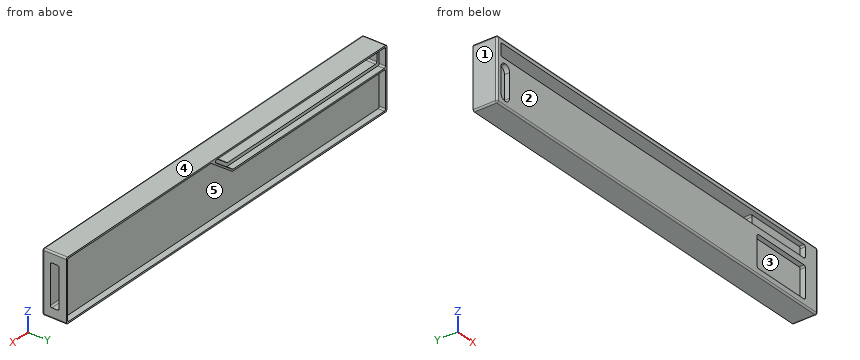
```python
from build123d import *

# Parameters (mm, degrees)
EXTRUDE_1_DEPTH     = 7.6
CUT_EXTRUDE_1_DEPTH = 2
CUT_EXTRUDE_2_DEPTH = 66.965312855
CUT_EXTRUDE_START   = -1.6
CUT_EXTRUDE_3_DEPTH = 1.6
CUT_EXTRUDE_START_2 = -3.3
CUT_EXTRUDE_4_DEPTH = 3.3
CUT_EXTRUDE_5_DEPTH = 10
FILLET_1_R          = 0.5


with BuildPart() as part:
    # Эскиз1 → Бобышка-Вытянуть1 (new body)
    with BuildSketch(Plane(origin=(0, 0, 0), x_dir=(1, 0, 0), z_dir=(0, 1, 0))):
        with BuildLine():
            Line((-64.5, 9.75), (64.5, 9.75))
            ThreePointArc((64.5, 9.75), (64.853553391, 9.603553391), (65, 9.25))
            Line((65, 9.25), (65, -9.25))
            ThreePointArc((65, -9.25), (64.853553391, -9.603553391), (64.5, -9.75))
            Line((64.5, -9.75), (-64.5, -9.75))
            ThreePointArc((-64.5, -9.75), (-64.853553391, -9.603553391), (-65, -9.25))
            Line((-65, -9.25), (-65, 9.25))
            ThreePointArc((-65, 9.25), (-64.853553391, 9.603553391), (-64.5, 9.75))
        make_face()
    extrude(amount=EXTRUDE_1_DEPTH)

    # Эскиз2 → Вырез-Вытянуть1 (cut)
    with BuildSketch(Plane(origin=(0, 7.6, 0), x_dir=(1, 0, 0), z_dir=(0, 1, 0))):
        with BuildLine():
            Line((-64, -3.25), (-2.666666667, -3.25))
            ThreePointArc((-2.666666667, -3.25), (-2.508552784, -3.275658351), (-2.366666667, -3.35))
            Line((-2.366666667, -3.35), (4.3, -8.35))
            ThreePointArc((4.3, -8.35), (4.474341649, -8.908113883), (4, -9.25))
            Line((4, -9.25), (-64, -9.25))
            ThreePointArc((-64, -9.25), (-64.353553391, -9.103553391), (-64.5, -8.75))
            Line((-64.5, -8.75), (-64.5, -3.75))
            ThreePointArc((-64.5, -3.75), (-64.353553391, -3.396446609), (-64, -3.25))
        make_face()
        with BuildLine():
            Line((-64, 9.25), (64, 9.25))
            ThreePointArc((64, 9.25), (64.353553391, 9.103553391), (64.5, 8.75))
            Line((64.5, 8.75), (64.5, -8.75))
            ThreePointArc((64.5, -8.75), (64.353553391, -9.103553391), (64, -9.25))
            Line((64, -9.25), (6.5, -9.25))
            ThreePointArc((6.5, -9.25), (6.341886117, -9.224341649), (6.2, -9.15))
            Line((6.2, -9.15), (-2.2, -2.85))
            ThreePointArc((-2.2, -2.85), (-2.341886117, -2.775658351), (-2.5, -2.75))
            Line((-2.5, -2.75), (-64, -2.75))
            ThreePointArc((-64, -2.75), (-64.353553391, -2.603553391), (-64.5, -2.25))
            Line((-64.5, -2.25), (-64.5, 8.75))
            ThreePointArc((-64.5, 8.75), (-64.353553391, 9.103553391), (-64, 9.25))
        make_face()
    extrude(amount=-CUT_EXTRUDE_1_DEPTH, mode=Mode.SUBTRACT)

    # Эскиз6 → Вырез-Вытянуть2 (cut, through all)
    with BuildSketch(Plane(origin=(0, 5.6, 0), x_dir=(1, 0, 0), z_dir=(0, 1, 0))):
        with BuildLine():
            Line((-63, -8.25), (1.020582083, -8.25))
            ThreePointArc((1.020582083, -8.25), (1.494923732, -7.908113883), (1.320582083, -7.35))
            Line((1.320582083, -7.35), (-2.695152274, -4.338199232))
            ThreePointArc((-2.695152274, -4.338199232), (-2.837038391, -4.263857583), (-2.995152274, -4.238199232))
            Line((-2.995152274, -4.238199232), (-63, -4.238199232))
            ThreePointArc((-63, -4.238199232), (-63.353553391, -4.384645841), (-63.5, -4.738199232))
            Line((-63.5, -4.738199232), (-63.5, -7.75))
            ThreePointArc((-63.5, -7.75), (-63.353553391, -8.103553391), (-63, -8.25))
        make_face()
    extrude(amount=-CUT_EXTRUDE_2_DEPTH, mode=Mode.SUBTRACT)

    # Эскиз7 → Вырез-Вытянуть3 (cut)
    with BuildSketch(Plane.XZ.offset(CUT_EXTRUDE_START)):
        with BuildLine():
            Line((-63, 4.25), (59.5, 4.25))
            ThreePointArc((59.5, 4.25), (59.853553391, 4.396446609), (60, 4.75))
            Line((60, 4.75), (60, 7.75))
            ThreePointArc((60, 7.75), (59.853553391, 8.103553391), (59.5, 8.25))
            Line((59.5, 8.25), (-63, 8.25))
            ThreePointArc((-63, 8.25), (-63.353553391, 8.103553391), (-63.5, 7.75))
            Line((-63.5, 7.75), (-63.5, 4.75))
            ThreePointArc((-63.5, 4.75), (-63.353553391, 4.396446609), (-63, 4.25))
        make_face()
        with BuildLine():
            Line((59.5, -7.75), (41, -7.75))
            ThreePointArc((41, -7.75), (40.646446609, -7.603553391), (40.5, -7.25))
            Line((40.5, -7.25), (40.5, 1.75))
            ThreePointArc((40.5, 1.75), (40.646446609, 2.103553391), (41, 2.25))
            Line((41, 2.25), (59.5, 2.25))
            ThreePointArc((59.5, 2.25), (59.853553391, 2.103553391), (60, 1.75))
            Line((60, 1.75), (60, -7.25))
            ThreePointArc((60, -7.25), (59.853553391, -7.603553391), (59.5, -7.75))
        make_face()
        with BuildLine():
            Line((-61.74, -8.15), (-61.76, -8.15))
            ThreePointArc((-61.76, -8.15), (-62.990365799, -7.640365799), (-63.5, -6.41))
            Line((-63.5, -6.41), (-63.5, 1.11))
            ThreePointArc((-63.5, 1.11), (-62.990365799, 2.340365799), (-61.76, 2.85))
            Line((-61.76, 2.85), (-61.74, 2.85))
            ThreePointArc((-61.74, 2.85), (-60.509634201, 2.340365799), (-60, 1.11))
            Line((-60, 1.11), (-60, -6.41))
            ThreePointArc((-60, -6.41), (-60.509634201, -7.640365799), (-61.74, -8.15))
        make_face()
    extrude(amount=CUT_EXTRUDE_3_DEPTH, mode=Mode.SUBTRACT)

    # Эскиз8 → Вырез-Вытянуть4 (cut)
    with BuildSketch(Plane.XZ.offset(-1.6).offset(CUT_EXTRUDE_START_2)):
        with BuildLine():
            Line((-63, 8.25), (40, 8.25))
            ThreePointArc((40, 8.25), (40.353553391, 8.103553391), (40.5, 7.75))
            Line((40.5, 7.75), (40.5, 4.75))
            ThreePointArc((40.5, 4.75), (40.353553391, 4.396446609), (40, 4.25))
            Line((40, 4.25), (-63, 4.25))
            ThreePointArc((-63, 4.25), (-63.353553391, 4.396446609), (-63.5, 4.75))
            Line((-63.5, 4.75), (-63.5, 7.75))
            ThreePointArc((-63.5, 7.75), (-63.353553391, 8.103553391), (-63, 8.25))
        make_face()
    extrude(amount=CUT_EXTRUDE_4_DEPTH, mode=Mode.SUBTRACT)

    # Эскиз9 → Вырез-Вытянуть5 (cut)
    with BuildSketch(Plane(origin=(65, 0, 0), x_dir=(0, 0, -1), z_dir=(1, 0, 0))):
        with BuildLine():
            Line((-6.05, 5.3), (6.05, 5.3))
            ThreePointArc((6.05, 5.3), (6.403553391, 5.153553391), (6.55, 4.8))
            Line((6.55, 4.8), (6.55, 3))
            ThreePointArc((6.55, 3), (6.403553391, 2.646446609), (6.05, 2.5))
            Line((6.05, 2.5), (-6.05, 2.5))
            ThreePointArc((-6.05, 2.5), (-6.403553391, 2.646446609), (-6.55, 3))
            Line((-6.55, 3), (-6.55, 4.8))
            ThreePointArc((-6.55, 4.8), (-6.403553391, 5.153553391), (-6.05, 5.3))
        make_face()
    extrude(amount=-CUT_EXTRUDE_5_DEPTH, mode=Mode.SUBTRACT)

    # Скругление1
    fillet_1_edges = [part.edges().sort_by_distance(p)[0] for p in [
        (0, 0, -9.75),
        (64.853553391, 0, -9.603553391),
        (65, 0, 0),
        (64.853553391, 0, 9.603553391),
        (0, 0, 9.75),
        (-64.853553391, 0, 9.603553391),
        (-65, 0, 0),
        (-64.853553391, 0, -9.603553391),
    ]]
    fillet(fillet_1_edges, radius=FILLET_1_R)


solid = part.part
```
Input: part model. Units: mm. Frame: model coordinates. Face numbers are marked on the shaded views. A direction names the side the tool comes from. Round coordinates to 2 decimals unless told otherwise and drop trailing zeros. Loops run counter-clockwise (first coordinate to the right, second up) from the corner with the lowest first, then second, coordinate; pieces in that order, holes last. Notation, with made-up numbers: (-13, -3) -> (4, -3) arc R24 cw to (4, 23) -> close; hole circle Ø9 at (-31.75, -29). An arc over 180 degrees is marked (long way). Use one line per item in the form item = value. Start each with the question number.
Item 1: Section query C-C on z = -3.5. Return the cut outline in (x, y).
Item 2: Section query B-B on x = -24. Return the cut outline in (y, z).
Item 3: Mould query, pull axis X, two halves, no side actions, for the marked faces 1, 2 and 3. Classes: pulls with the +X half, pulls with the -X half, needs draft (parallel to the pull), parting line crosses it, or undercut.
Item 4: Section query A-A on x = 57. Return the cut outline in (y, z), then the cut area to 3 significant figures.
Item 5: Contact query for flat-ended pins moving along their axis: pin 1 Ø11 at (x, z) = (55, -4) entering from -Y; pin 2 Ø5 at (x, z) = (60.5, -3) entering from +Y. Output: stop coordinate, or through.
Item 6: Material intervals for L1, parallel to Z at x = -5.5, y = 6.5; L2, parallel to X at y = 0.5, z = -6.25; L3, parallel to Z at x = -20, y = 5.25, sorted ascending. Write a range as from..to.
Item 7: Section query D-D on x = 36. Return the cut outline in (y, z).
Item 8: Set-up query: the marked faces 4 and 5. Return all of +Z, -Z, +X, -X, +Y, -Y with unobstructed straight access to the full face (end or side cutting, diameter ignored); none if empty.
Ans:
q1.outline = (-65, 0.5) arc R0.5 ccw to (-64.5, 0) -> (-63.5, 0) -> (-63.5, 1.6) -> (-60, 1.6) -> (-60, 0) -> (40.5, 0) -> (40.5, 1.6) -> (60, 1.6) -> (60, 0) -> (64.5, 0) arc R0.5 ccw to (65, 0.5) -> (65, 2.5) -> (55, 2.5) -> (55, 5.3) -> (65, 5.3) -> (65, 7.6) -> (64.5, 7.6) -> (64.5, 5.6) -> (-64.5, 5.6) -> (-64.5, 7.6) -> (-65, 7.6) -> close
q2.outline = (0, -9.25) arc R0.5 ccw to (0.5, -9.75) -> (7.6, -9.75) -> (7.6, -9.25) -> (5.6, -9.25) -> (5.6, 2.75) -> (7.6, 2.75) -> (7.6, 3.25) -> (5.6, 3.25) -> (5.6, 4.24) -> (0, 4.24) -> close; (0, 8.25) -> (5.6, 8.25) -> (5.6, 9.25) -> (7.6, 9.25) -> (7.6, 9.75) -> (0.5, 9.75) arc R0.5 ccw to (0, 9.25) -> close
q3.face_1 = pulls with the -X half
q3.face_2 = needs draft
q3.face_3 = undercut
q4.outline = (0, -9.25) arc R0.5 ccw to (0.5, -9.75) -> (7.6, -9.75) -> (7.6, -9.25) -> (5.6, -9.25) -> (5.6, 9.25) -> (7.6, 9.25) -> (7.6, 9.75) -> (0.5, 9.75) arc R0.5 ccw to (0, 9.25) -> (0, 8.25) -> (1.6, 8.25) -> (1.6, 4.25) -> (0, 4.25) -> (0, 2.25) -> (1.6, 2.25) -> (1.6, -7.75) -> (0, -7.75) -> close; hole (2.5, -6.05) arc R0.5 ccw to (3, -6.55) -> (4.8, -6.55) arc R0.5 ccw to (5.3, -6.05) -> (5.3, 6.05) arc R0.5 ccw to (4.8, 6.55) -> (3, 6.55) arc R0.5 ccw to (2.5, 6.05) -> close
q4.area = 52.2 mm^2
q5.pin_1 = 0
q5.pin_2 = 5.6
q6.L1 = -9.75..-9.25, 2.75..3.25, 9.25..9.75
q6.L2 = -65..-63.5, -60..40.5, 60..65
q6.L3 = -9.75..4.24, 8.25..9.75
q7.outline = (0, -9.25) arc R0.5 ccw to (0.5, -9.75) -> (7.6, -9.75) -> (7.6, -9.25) -> (5.6, -9.25) -> (5.6, 9.25) -> (7.6, 9.25) -> (7.6, 9.75) -> (0.5, 9.75) arc R0.5 ccw to (0, 9.25) -> (0, 8.25) -> (4.9, 8.25) -> (4.9, 4.25) -> (0, 4.25) -> close
q8.face_4 = +Z, +X, -X, +Y, -Y
q8.face_5 = +Y
